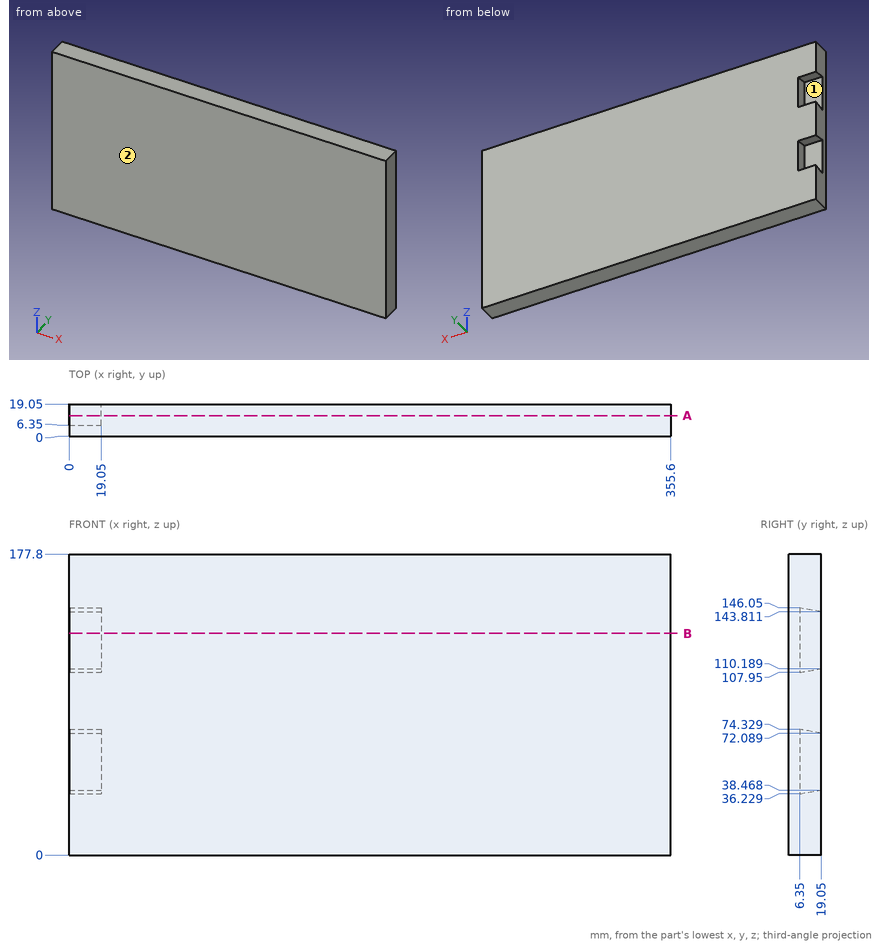
Drawing for the job (mm, zero at the part's lowest x, y, z). Round coordinates to 2 decimals unless told otherwise and drop trailing zeros. Write each loop counter-clockwise with the first axis right and the second up, starting at its lowest first coordinate (ties: lowest second). Pieces come first, ordered by that corner, then holes. Notation, with made-up numbers: (89, 0) - (131, 0) arc R17 ccw to (131, 26) - close; hole circle Ø7 at (66, 61.25). An arc over 180 degrees is marked (long way). Return JSON: item names as keys, results as strings. Group by question number.
Item 1: Probe probe 1 along Z at (x, y) = (16, 9.75); probe 2 along X at (y, z) = (7, 139.5). List the from-to ranges inside material, lowest first.
Item 2: Flat gauge pin, fed straight in: pin 1 Ø5.5 at (x, z) = (8, 56.5) entering from +Y. Where does the tip first touch, or does it go through?
Item 3: Band-saw the part on A-A on y = 12.25. List the corners of the cut face in (x, z), plus the area to 3 significant figures.
Item 4: Band-saw the part on B-B on z = 131. List the corners of the cut face in (x, y), plus the area to 3 significant figures.
Item 5: Mould opens along Z. For the marked faces 1 and 2 say: +Z half, -Z half, draft (parallel to the pull), parting line (faces both ways), or undercut.
Resolved:
{
 "1": {"probe 1": "z = 0 to 36.83, 73.73 to 108.55, 145.45 to 177.8", "probe 2": "x = 19.05 to 355.6"},
 "2": {"pin 1": "stops at y = 6.35"},
 "3": {"outline": "(0, 0) - (355.6, 0) - (355.6, 177.8) - (0, 177.8) - (0, 145.01) - (19.05, 145.01) - (19.05, 108.99) - (0, 108.99) - (0, 73.29) - (19.05, 73.29) - (19.05, 37.27) - (0, 37.27) - close", "area": "61,900 mm²"},
 "4": {"outline": "(0, 0) - (355.6, 0) - (355.6, 19.05) - (19.05, 19.05) - (19.05, 6.35) - (0, 6.35) - close", "area": "6,530 mm²"},
 "5": {"face 1": "undercut", "face 2": "draft"}
}
